from build123d import *

# Parameters (mm, degrees)
BASE_FLANGE1_DEPTH = 16
SKETCH6_W          = 1.6
SKETCH6_H          = 10.2
CUT_EXTRUDE1_DEPTH = 10
SKETCH7_R          = 3
CUT_EXTRUDE2_DEPTH = 10
CUT_EXTRUDE3_DEPTH = 10
FILLET1_R          = 0.2
SKETCH11_R         = 1.55
TAB1_DEPTH         = 1.5
SKETCH15_R         = 1.6
CUT_EXTRUDE6_DEPTH = 10
SKETCH9_R          = 3.025
SKETCH9_R_2        = 1.5
CUT_EXTRUDE4_DEPTH = 10


# Sheet-metal steps are written as plain solids
with BuildPart() as part:
    # Sketch1 → Base-Flange1 (new body)
    with BuildSketch(Plane(origin=(0, 0, 0), x_dir=(1, 0, 0), z_dir=(0, 1, 0))):
        with BuildLine():
            Line((65.5, 50), (65.5, 3.5))
            ThreePointArc((65.5, 3.5), (64.474873734, 1.025126266), (62, 0))
            Line((62, 0), (3.5, 0))
            ThreePointArc((3.5, 0), (1.025126266, 1.025126266), (0, 3.5))
            Line((0, 3.5), (0, 53))
            Line((0, 53), (1.5, 53))
            Line((1.5, 53), (1.5, 3.5))
            ThreePointArc((1.5, 3.5), (2.085786438, 2.085786438), (3.5, 1.5))
            Line((3.5, 1.5), (62, 1.5))
            ThreePointArc((62, 1.5), (63.414213562, 2.085786438), (64, 3.5))
            Line((64, 3.5), (64, 50))
            Line((64, 50), (65.5, 50))
        make_face()
    extrude(amount=BASE_FLANGE1_DEPTH)

    # Sketch6 → Cut-Extrude1 (cut)
    with BuildSketch(Plane(origin=(0, 0, -1.5), x_dir=(-1, 0, 0), z_dir=(0, 0, -1))):
        with Locations((-25.8, 8)):
            Rectangle(SKETCH6_W, SKETCH6_H)
    extrude(amount=-CUT_EXTRUDE1_DEPTH, mode=Mode.SUBTRACT)

    # Sketch7 → Cut-Extrude2 (cut)
    with BuildSketch(Plane(origin=(65.5, 0, 0), x_dir=(0, 0, -1), z_dir=(1, 0, 0))):
        with Locations((35.5, 8)):
            Circle(SKETCH7_R)
    extrude(amount=-CUT_EXTRUDE2_DEPTH, mode=Mode.SUBTRACT)

    # Sketch8 → Cut-Extrude3 (cut)
    with BuildSketch(Plane(origin=(65.5, 0, 0), x_dir=(0, 0, -1), z_dir=(1, 0, 0))):
        Polygon((50, 16), (44.7, 16), (44.7, 13), (46.5, 13), (46.5, 3), (44.7, 3), (44.7, 0), (50, 0), (53, 0), (53, 16), align=None)
    extrude(amount=-CUT_EXTRUDE3_DEPTH, mode=Mode.SUBTRACT)

    # Fillet1
    fillet1_edges = [part.edges().sort_by_distance(p)[0] for p in [
        (0.75, 0, -53),
        (0.75, 16, -53),
        (64.75, 16, -44.7),
        (64.75, 0, -44.7),
        (64.75, 3, -46.5),
        (64.75, 13, -46.5),
    ]]
    fillet(fillet1_edges, radius=FILLET1_R)

    # Sketch11 → Tab1 (add)
    with BuildSketch(Plane(origin=(65.5, 0, 0), x_dir=(0, 0, -1), z_dir=(1, 0, 0))):
        with BuildLine():
            Line((46.5, 12.8), (52.5, 12.8))
            ThreePointArc((52.5, 12.8), (52.853553391, 12.653553391), (53, 12.3))
            Line((53, 12.3), (53, 3.7))
            ThreePointArc((53, 3.7), (52.853553391, 3.346446609), (52.5, 3.2))
            Line((52.5, 3.2), (46.5, 3.2))
            Line((46.5, 3.2), (46.5, 12.8))
        make_face()
        with Locations((49.9, 8)):
            Circle(SKETCH11_R, mode=Mode.SUBTRACT)
    extrude(amount=-TAB1_DEPTH)

    # Sketch15 → Cut-Extrude6 (cut)
    with BuildSketch(Plane.XY):
        with Locations((35.5, 8)):
            Circle(SKETCH15_R)
        with Locations((53.5, 8)):
            Circle(SKETCH15_R)
        with Locations((11.5, 8)):
            Circle(SKETCH15_R)
    extrude(amount=-CUT_EXTRUDE6_DEPTH, mode=Mode.SUBTRACT)

    # Sketch9 → Cut-Extrude4 (cut)
    with BuildSketch(Plane(origin=(1.5, 0, 0), x_dir=(0, 0, -1), z_dir=(1, 0, 0))):
        with Locations((35.5, 8)):
            Circle(SKETCH9_R)
        with Locations((30.5, 3)):
            Circle(SKETCH9_R_2)
        with Locations((46, 11)):
            Circle(SKETCH9_R_2)
    extrude(amount=-CUT_EXTRUDE4_DEPTH, mode=Mode.SUBTRACT)


solid = part.part
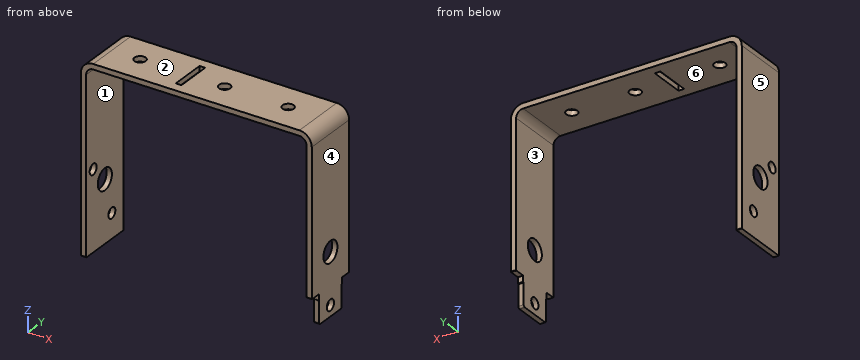
Verification items for the finished model (mm, model axes). Face numbers are marked on the shaded views. A direction names the side the tool comes from. Round coordinates to 2 decimals unless told otherwise and drop trailing zeros. Order: outer loops, then holes, each group sorted by start corner. A loop starts at its lowest first (then second) coordinate and runs counter-clockwise, first axis right, second up.
1. Access from +Z, -Z, +X, -X, +Y, -Y to the whole of each face (thin tool, end or side, straight path). Record for the marked faces 1 and 2.
Final values:
face 1: -Z, +Y, -Y
face 2: +Z, +X, -X, +Y, -Y
2. Section check A-A on z = -49.9. Record the cut outline in (x, y).
Final values:
outline: (0, 0) - (1.5, 0) - (1.5, 16) - (0, 16) - close; (64, 3.2) - (65.5, 3.2) - (65.5, 6.45) - (64, 6.45) - close; (64, 9.55) - (65.5, 9.55) - (65.5, 12.8) - (64, 12.8) - close
3. Section check B-B on x = 35.5. Record the cut outline in (y, z), then the cut area to 3 significant figures.
Final values:
outline: (0, -1.5) - (6.4, -1.5) - (6.4, 0) - (0, 0) - close; (9.6, -1.5) - (16, -1.5) - (16, 0) - (9.6, 0) - close
area: 19.2 mm2
4. Section check C-C on z = -15.5. Record the cut outline in (x, y), then the cut area to 3 significant figures.
Final values:
outline: (0, 0) - (1.5, 0) - (1.5, 16) - (0, 16) - close; (64, 0) - (65.5, 0) - (65.5, 16) - (64, 16) - close
area: 48.0 mm2
5. Go/stop test with flat-tipped pins: P1, Ø1.2, axis at y = 5.5, z = -1, coming from the +X side; P2, Ø8, axis at x = 36, y = 11, coming from the -Z side; P3, Ø1.2, axis at x = 64.5, z = -50.5, coming from the -Y side; P4, Ø12, axis at x = 57.5, z = -41.5, coming from the +Y side. Record where each tip stops, or that it passes through.
Final values:
P1: stops at x = 64.94
P2: stops at z = -1.5
P3: stops at y = 3.2
P4: passes through
6. Thickness scan on L1, parallel to X at y = 11.5, z = -29; L2, parallel to Y at x = 65, z = -35.5; L3, parallel to Y at x = 64.9, z = -49.9. Record the ranges inside material, lowest first.
Final values:
L1: x = 0 to 1.5, 64 to 65.5
L2: y = 0 to 5, 11 to 16
L3: y = 3.2 to 6.45, 9.55 to 12.8
7. Release check for a two-part mould opening along X. For the marked faces 3, 4, 5 and 6 record: +X half, -X half, draft (parallel to the pull), parting line (faces both ways), or undercut.
Final values:
face 3: undercut
face 4: +X half
face 5: -X half
face 6: undercut
8. Section check D-D on y = 8. State how many separate pieces and enclosed holes the cut face has, then the cut area to 3 significant figures.
Final values:
separate pieces: 8
enclosed holes: 0
area: 210 mm2
